The model under review builds one solid part; all positions refer to its coordinate system, in mm. Face numbers are marked on the shaded views. A direction names the side the tool comes from. Give positions to 0.01 mm unless a question says otherwise; leave off trailing zeros. Order: outer loops, then holes, each group sorted by start corner. A loop starts at its lowest first (then second) coordinate and runs counter-clockwise, first axis right, second up. Notation, with made-up numbers: (13, -10.75) -> (44, -10.75) arc R32 ccw to (44, 24.25) -> close; hole circle Ø7 at (12.25, 0.5). An arc over 180 degrees is marked (long way). Use one line per item in the form item = value.
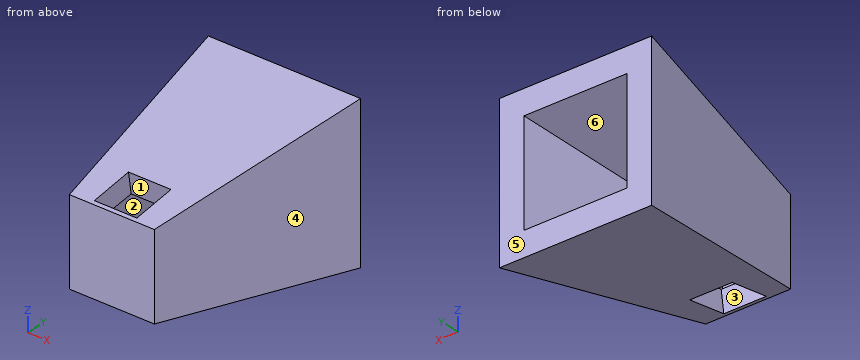
```python
from build123d import *

# Parameters (mm, degrees)
SKETCH1_W           = 50.8
SKETCH1_H           = 50.8
BOSS_EXTRUDE1_DEPTH = 127
BOSS_EXTRUDE1_DRAFT = -9
SKETCH2_W           = 61.565647843
SKETCH2_H           = 61.565647842
CUT_EXTRUDE1_DEPTH  = 124.46
CUT_EXTRUDE1_DRAFT  = -8
CUT_EXTRUDE2_REACH  = 165.697
SKETCH3_W           = 25.4
SKETCH3_H           = 25.4
CUT_EXTRUDE3_REACH  = 161.627
SKETCH4_W           = 25.4
SKETCH4_H           = 25.4


with BuildPart() as part:
    # Sketch1 → Boss-Extrude1 (with draft: the straight prism first)
    with BuildSketch(Plane(origin=(0, 0, 0), x_dir=(1, 0, 0), z_dir=(0, 1, 0))):
        with Locations((-18.114225515, -17.77595618)):
            Rectangle(SKETCH1_W, SKETCH1_H)
    extrude(amount=BOSS_EXTRUDE1_DEPTH)
    # Boss-Extrude1: the draft: its side faces are tilted about the plane it starts from
    boss_extrude1_sides = [part.faces().sort_by_distance(p)[0] for p in [
        (-43.514225515, 63.5, 17.77595618),
        (-18.114225515, 63.5, 43.17595618),
        (7.285774485, 63.5, 17.77595618),
        (-18.114225515, 63.5, -7.62404382),
    ]]
    draft(boss_extrude1_sides, Plane(origin=(0, 0, 0), x_dir=(1, 0, 0), z_dir=(0, 1, 0)), BOSS_EXTRUDE1_DRAFT)


with BuildPart() as cut_extrude1_tool:
    # Sketch2 → Cut-Extrude1 (with draft: the straight prism first)
    with BuildSketch(Plane(origin=(0, 127, 0), x_dir=(1, 0, 0), z_dir=(0, 1, 0))):
        with Locations((-18.114225515, -17.77595618)):
            Rectangle(SKETCH2_W, SKETCH2_H)
    extrude(amount=-CUT_EXTRUDE1_DEPTH)
    # Cut-Extrude1: the draft: its side faces are tilted about the plane it starts from
    cut_extrude1_sides = [cut_extrude1_tool.faces().sort_by_distance(p)[0] for p in [
        (-48.897049437, 64.77, 17.77595618),
        (-18.114225515, 64.77, 48.558780101),
        (12.668598406, 64.77, 17.77595618),
        (-18.114225515, 64.77, -13.006867741),
    ]]
    draft(cut_extrude1_sides, Plane(origin=(0, 127, 0), x_dir=(1, 0, 0), z_dir=(0, 1, 0)), CUT_EXTRUDE1_DRAFT)


with BuildPart() as part_1:
    add(part.part)

    # Cut-Extrude1: cut by cut_extrude1_tool
    add(cut_extrude1_tool.part, mode=Mode.SUBTRACT)

    # Cut-Extrude2: up to this plane
    cut_extrude2_end = Plane(origin=(-48.897049437, 127, 48.558780101), z_dir=(0, -0.1391731009600655, 0.9902680687415704))
    # Sketch3 → Cut-Extrude2 (cut, up to the surface)
    with BuildSketch(Plane(origin=(0, -6.671052104, 42.119365326), x_dir=(1, 0, 0), z_dir=(0, -0.15643446504023092, 0.9876883405951379)), mode=Mode.PRIVATE) as cut_extrude2_sk1:
        with Locations((-17.909049437, 21.994207608)):
            Rectangle(SKETCH3_W, SKETCH3_H)
    cut_extrude2_tool1 = split(extrude(cut_extrude2_sk1.sketch, amount=-CUT_EXTRUDE2_REACH, mode=Mode.PRIVATE), bisect_by=cut_extrude2_end, keep=Keep.BOTH, mode=Mode.PRIVATE)
    add(cut_extrude2_tool1.solids().sort_by_distance((-17.909049, 15.05237, 45.560017))[0], mode=Mode.SUBTRACT)

    # Cut-Extrude3: up to this plane
    cut_extrude3_end = Plane(origin=(-48.897049437, 127, -13.006867741), z_dir=(0, -0.1391731009600655, -0.9902680687415704))
    # Sketch4 → Cut-Extrude3 (cut, up to the surface)
    with BuildSketch(Plane(origin=(0, -1.177979553, -7.437470188), x_dir=(-1, 0, 0), z_dir=(0, -0.15643446504023092, -0.9876883405951379)), mode=Mode.PRIVATE) as cut_extrude3_sk1:
        with Locations((18.319401594, 16.432663216)):
            Rectangle(SKETCH4_W, SKETCH4_H)
    cut_extrude3_tool1 = split(extrude(cut_extrude3_sk1.sketch, amount=-CUT_EXTRUDE3_REACH, mode=Mode.PRIVATE), bisect_by=cut_extrude3_end, keep=Keep.BOTH, mode=Mode.PRIVATE)
    add(cut_extrude3_tool1.solids().sort_by_distance((-18.319402, 15.05237, -10.008105))[0], mode=Mode.SUBTRACT)


solid = part_1.part
```
1. For L1, parallel to Z at x = -9.5, y = 103.5; L2, parallel to X at y = 27, z = 45.5; L3, parallel to X at y = 49, z = 30.5, list the stretches that pass through material, from the lowest coordinate up.
Values:
L1 = -24.02 to -9.7, 45.26 to 59.57
L2 = -47.79 to -30.61, -5.21 to 11.56
L3 = -51.28 to -37.93, 1.71 to 15.05
2. Add section A-A on x = -25.5. Give the boundary of the cut face in (y, z), then the cut area to 3 significant figures.
Values:
outline = (0, -7.62) -> (2.51, -8.02) -> (4.45, 4.22) -> (2.54, 4.48) -> (2.54, 31.07) -> (4.45, 31.34) -> (2.51, 43.57) -> (0, 43.18) -> close; (27.6, -11.99) -> (127, -27.74) -> (127, -13.01) -> (29.6, 0.68) -> close; (27.6, 47.55) -> (29.6, 34.87) -> (127, 48.56) -> (127, 63.29) -> close
area = 2,880 mm^2
3. Add section D-D on y = 14. Give the boundary of the cut face in (x, z).
Values:
outline = (-45.73, -9.84) -> (-31.02, -9.84) -> (-31.02, 2.87) -> (-33.02, 2.87) -> (-33.02, 32.68) -> (-30.61, 32.68) -> (-30.61, 45.39) -> (-45.73, 45.39) -> close; (-5.62, -9.84) -> (9.5, -9.84) -> (9.5, 45.39) -> (-5.21, 45.39) -> (-5.21, 32.68) -> (-3.21, 32.68) -> (-3.21, 2.87) -> (-5.62, 2.87) -> close
4. Tool access review of the marked faces 1, 2 and 3: name each direction out of +Z, -Z, +X, -X, +Y, -Y from which nothing blocks a thin tool from reaching the whole face with its end or side.
Values:
face_1 = none
face_2 = +Y
face_3 = -Z
5. For pin 1 Ø5 at (y, z) = (50, 21) entering from -X; pin 2 Ø18 at (y, z) = (19, 38.5) entering from -X; pin 3 Ø13 at (y, z) = (14, -5) entering from -X, all flat-tipped, find the tip position at first contact; note any pin that passes through.
Values:
pin_1 = -51.83
pin_2 = -47.95
pin_3 = -46.76
6. Add section C-C on y = 60. Give the boundary of the cut face in (x, z), then the cut area to 3 significant figures.
Values:
outline = (-53.02, -17.13) -> (16.79, -17.13) -> (16.79, 52.68) -> (-53.02, 52.68) -> close; hole (-39.48, -3.59) -> (3.25, -3.59) -> (3.25, 39.14) -> (-39.48, 39.14) -> close
area = 3,050 mm^2
7. The part is to be moulded in two halves that separate along X. For the marked faces 4, 5 and 6, say which applies: +X half, -X half, draft (parallel to the pull), parting line (faces both ways), or undercut.
Values:
face_4 = +X half
face_5 = draft
face_6 = undercut
8. Add section B-B on z = 14.5. Give the boundary of the cut face in (x, y), then the cut area to 3 significant figures.
Values:
outline = (-63.63, 127) -> (-43.51, 0) -> (7.29, 0) -> (27.4, 127) -> (12.67, 127) -> (-4.82, 2.54) -> (-31.41, 2.54) -> (-48.9, 127) -> close
area = 3,520 mm^2
